For this review, take the finished solid that the model builds, in its own axes (mm). A direction names the side the tool comes from. Round coordinates to 2 decimals unless told otherwise and drop trailing zeros. Write each loop counter-clockwise with the first axis right and the second up, starting at its lowest first coordinate (ties: lowest second). Pieces come first, ordered by that corner, then holes.
from build123d import *

# Parameters (mm, degrees)
SKETCH1_W           = 73.8
SKETCH1_H           = 38.8
SKETCH1_W_2         = 71.4
SKETCH1_H_2         = 36.4
BOSS_EXTRUDE1_DEPTH = 1.8
SKETCH1_3_W         = 73.8
SKETCH1_3_H         = 38.8
SKETCH1_3_W_2       = 71.4
SKETCH1_3_H_2       = 36.4
BOSS_EXTRUDE2_DEPTH = 18
SKETCH2_W           = 34.8
SKETCH2_H           = 10.5
CUT_EXTRUDE1_DEPTH  = 1.2


with BuildPart() as part:
    # Sketch1 → Boss-Extrude1 (new body)
    with BuildSketch(Plane(origin=(0, 0, 0), x_dir=(1, 0, 0), z_dir=(0, 1, 0))):
        Rectangle(SKETCH1_W, SKETCH1_H)
        Rectangle(SKETCH1_W_2, SKETCH1_H_2, mode=Mode.SUBTRACT)
        Rectangle(SKETCH1_W_2, SKETCH1_H_2)
    extrude(amount=BOSS_EXTRUDE1_DEPTH)

    # Sketch1<3> → Boss-Extrude2 (add)
    with BuildSketch(Plane(origin=(0, 0, 0), x_dir=(1, 0, 0), z_dir=(0, 1, 0))):
        Rectangle(SKETCH1_3_W, SKETCH1_3_H)
        Rectangle(SKETCH1_3_W_2, SKETCH1_3_H_2, mode=Mode.SUBTRACT)
    extrude(amount=BOSS_EXTRUDE2_DEPTH)

    # Sketch2 → Cut-Extrude1 (cut)
    with BuildSketch(Plane(origin=(36.9, 0, 0), x_dir=(0, 0, -1), z_dir=(1, 0, 0))):
        with Locations((0, 9.25)):
            Rectangle(SKETCH2_W, SKETCH2_H)
    extrude(amount=-CUT_EXTRUDE1_DEPTH, mode=Mode.SUBTRACT)


solid = part.part
(1) We need section A-A, the plane z = 2. Give the boundary of the cut face in (x, y), and give its area (3 significant figures).
Geometry check:
outline: (-36.9, 0) - (36.9, 0) - (36.9, 4) - (35.7, 4) - (35.7, 1.8) - (-35.7, 1.8) - (-35.7, 18) - (-36.9, 18) - close; (35.7, 14.5) - (36.9, 14.5) - (36.9, 18) - (35.7, 18) - close
area: 159 mm2
(2) We need section C-C, the plane y = 10. Give the boundary of the cut face in (x, z).
Geometry check:
outline: (-36.9, -19.4) - (36.9, -19.4) - (36.9, -17.4) - (35.7, -17.4) - (35.7, -18.2) - (-35.7, -18.2) - (-35.7, 18.2) - (35.7, 18.2) - (35.7, 17.4) - (36.9, 17.4) - (36.9, 19.4) - (-36.9, 19.4) - close
(3) Mouldability with a two-part tool opening along X and no side actions: class faces 1 (the face through (0, 10, 18.2)), 2 (the face through (-11, 18, -19)), 3 (the face through (36.9, 15, 0)), 4 (the face through (35.7, 15, 1)) as pulls with the +X half, pulls with the -X half, needs draft (parallel to the pull), parting line crosses it, or undercut.
Geometry check:
face 1: undercut
face 2: needs draft
face 3: pulls with the +X half
face 4: undercut
(4) For pin 1 Ø6 at (x, z) = (-16.5, -13.5) entering from +Y, flat-tipped, find the tip position at first contact; note if it passes through.
Geometry check:
pin 1: stops at y = 1.8
(5) For faces 5 (the face through (-35.7, 10, 0)), 6 (the face through (-1, 0, 0)), list the 3-axis set-ups (+Z, -Z, +X, -X, +Y, -Y) from which the entire face can be reached by the end or side of a thin tool; tool diameter is ignored.
Geometry check:
face 5: +Y
face 6: +Z, -Z, +X, -X, -Y
(6) For line 1 along Z through (x, y) = (-23, 9); line 2 along X through (y, z) = (15.5, 1); line 3 along Y through (x, z) = (-11, 7), list the stretches that pass through material, from the lowest coordinate up.
Geometry check:
line 1: z = -19.4 to -18.2, 18.2 to 19.4
line 2: x = -36.9 to -35.7, 35.7 to 36.9
line 3: y = 0 to 1.8
(7) We need section B-B, the plane x = -5. Give the boundary of the cut face in (y, z).
Geometry check:
outline: (0, -19.4) - (18, -19.4) - (18, -18.2) - (1.8, -18.2) - (1.8, 18.2) - (18, 18.2) - (18, 19.4) - (0, 19.4) - close
